Check sheet for the modelled part. Datum: model origin and axes. Units: mm. Give positions to 0.01 mm unless a question says otherwise; leave off trailing zeros. Write each loop counter-clockwise with the first axis right and the second up, starting at its lowest first coordinate (ties: lowest second). Pieces come first, ordered by that corner, then holes. Notation, with made-up numbers: M 30,38 L 69,38 A19 cw 69,74 Z; hole C -17,-5 d6. An arc over 180 degrees is marked long. One line per item, written item: value. Start each with the question number.
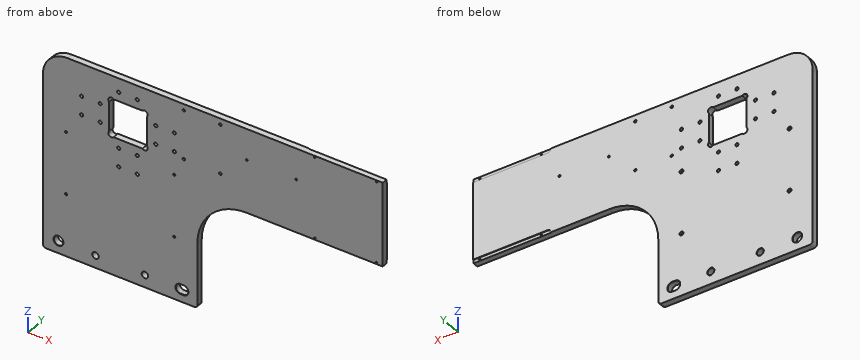
from build123d import *

# Parameters (mm, degrees)
SKETCH1_W                                      = 317.5
SKETCH1_H                                      = 406.4
BOSS_EXTRUDE1_DEPTH                            = 12.7
FILLET1_R                                      = 6.35
F_3_4_START                                    = 123.825
F_3_4_0_7500_DOWEL_SLOT1_3_DEPTH               = 6.35
F_1_2_CLEARANCE_HOLE1_D                        = 13.49248
F_1_2_CLEARANCE_HOLE1_CSINK_D                  = 14.76248
F_1_2_CLEARANCE_HOLE1_CSINK_ANGLE              = 90
SKETCH8_W                                      = 381
SKETCH8_H                                      = 171.45
BOSS_EXTRUDE2_DEPTH                            = 12.7
FILLET2_R                                      = 50.8
FILLET3_R                                      = 101.6
F_1_8_0_1250_DOWEL_HOLE1_D                     = 3.175
F_1_8_0_1250_DOWEL_HOLE1_CSINK_D               = 4.445
F_1_8_0_1250_DOWEL_HOLE1_CSINK_ANGLE           = 90
CUT_EXTRUDE1_DEPTH                             = 577.872249723
F_5_16_18_TAPPED_HOLE1_D                       = 6.5278
F_5_16_18_TAPPED_HOLE1_DEPTH                   = 20.1168
F_5_16_18_TAPPED_HOLE1_TIP                     = 1.961148974
CBORE_FOR_8_SOCKET_HEAD_CAP_SCREW1_D           = 4.4958
CBORE_FOR_8_SOCKET_HEAD_CAP_SCREW1_CBORE_D     = 7.9375
CBORE_FOR_8_SOCKET_HEAD_CAP_SCREW1_CBORE_DEPTH = 4.1656
SKETCH23_W                                     = 160.02
SKETCH23_H                                     = 6.858
CUT_EXTRUDE3_DEPTH                             = 1.27
FILLET4_R                                      = 6.35
F_10_32_TAPPED_HOLE1_D                         = 4.0386
F_1_4_20_TAPPED_HOLE1_D                        = 5.1054


with BuildPart() as part:
    # Sketch1 → Boss-Extrude1 (new body)
    with BuildSketch(Plane(origin=(0, 0, 0), x_dir=(1, 0, 0), z_dir=(0, 1, 0))):
        Rectangle(SKETCH1_W, SKETCH1_H)
    extrude(amount=BOSS_EXTRUDE1_DEPTH)

    # Fillet1
    fillet1_edges = [part.edges().sort_by_distance(p)[0] for p in [
        (-158.75, 6.35, -203.2),
        (158.75, 6.35, -203.2),
    ]]
    fillet(fillet1_edges, radius=FILLET1_R)

    # Sketch3 → 3/4 (0.7500) Dowel Hole1 (revolve, cut)
    with BuildSketch(Plane(origin=(-127, 12.7, -177.8), x_dir=(0, 0, 1), z_dir=(1, 0, 0))):
        Polygon((0, 0), (0, 12.7), (10.16, 12.7), (9.525, 12.065), (9.525, 0.635), (10.16, 0), align=None)
    revolve(axis=Axis((-127, 19.05, -177.8), (0, -1, 0)), mode=Mode.SUBTRACT)

    # 3/4 (0.7500) Dowel Slot1: read off the stored shape, not the designer's step
    # 3/4 (0.7500) Dowel Slot1 outline → 3/4 (0.7500) Dowel Slot1 (revolve, cut)
    with BuildSketch(Plane(origin=(130.175, 0, -177.8), x_dir=(1, 0, 0), z_dir=(0, 0, 1))):
        Polygon((0, 0), (10.16, 0), (9.525, 0.635), (9.525, 12.065), (10.16, 12.7), (0, 12.7), align=None)
    revolve(axis=Axis((130.175, 0, -177.8), (0, 1, 0)), mode=Mode.SUBTRACT)

    # 3_4 _0.7500_ Dowel Slot1 2 outline → 3_4 _0.7500_ Dowel Slot1 2 (revolve, cut)
    with BuildSketch(Plane(origin=(123.825, 0, -177.8), x_dir=(1, 0, 0), z_dir=(0, 0, 1))):
        Polygon((0, 0), (10.16, 0), (9.525, 0.635), (9.525, 12.065), (10.16, 12.7), (0, 12.7), align=None)
    revolve(axis=Axis((123.825, 0, -177.8), (0, 1, 0)), mode=Mode.SUBTRACT)

    # 3_4 _0.7500_ Dowel Slot1 3 outline → 3_4 _0.7500_ Dowel Slot1 3 (cut)
    with BuildSketch(Plane.YZ.offset(F_3_4_START)):
        Polygon((0.635, -187.325), (12.065, -187.325), (12.7, -187.96), (12.7, -167.64), (12.065, -168.275), (0.635, -168.275), (0, -167.64), (0, -187.96), align=None)
    extrude(amount=F_3_4_0_7500_DOWEL_SLOT1_3_DEPTH, mode=Mode.SUBTRACT)

    # 1/2 Clearance Hole1 (through all)
    with Locations(Plane(origin=(0, 12.7, 0), x_dir=(1, 0, 0), z_dir=(0, 1, 0))):
        with Locations((-50.8, 177.8), (50.8, 177.8)):
            CounterSinkHole(F_1_2_CLEARANCE_HOLE1_D / 2, F_1_2_CLEARANCE_HOLE1_CSINK_D / 2, counter_sink_angle=F_1_2_CLEARANCE_HOLE1_CSINK_ANGLE)

    # Sketch8 → Boss-Extrude2 (add)
    with BuildSketch(Plane(origin=(0, 0, 0), x_dir=(1, 0, 0), z_dir=(0, 1, 0))):
        with Locations((349.25, -117.475)):
            Rectangle(SKETCH8_W, SKETCH8_H)
    extrude(amount=BOSS_EXTRUDE2_DEPTH)

    # Fillet2
    fillet2_edges = [part.edges().sort_by_distance(p)[0] for p in [
        (-158.75, 6.35, 203.2),
    ]]
    fillet(fillet2_edges, radius=FILLET2_R)

    # Fillet3
    fillet3_edges = [part.edges().sort_by_distance(p)[0] for p in [
        (158.75, 6.35, 31.75),
    ]]
    fillet(fillet3_edges, radius=FILLET3_R)

    # 1/8 (0.1250) Dowel Hole1 (through all)
    with Locations(Plane(origin=(0, 12.7, 0), x_dir=(1, 0, 0), z_dir=(0, 1, 0))):
        with Locations((400.05, -34.925), (527.05, -34.925), (400.05, -200.025), (527.05, -200.025)):
            CounterSinkHole(F_1_8_0_1250_DOWEL_HOLE1_D / 2, F_1_8_0_1250_DOWEL_HOLE1_CSINK_D / 2, counter_sink_angle=F_1_8_0_1250_DOWEL_HOLE1_CSINK_ANGLE)

    # Sketch13 → Cut-Extrude1 (cut, through all)
    with BuildSketch(Plane(origin=(0, 12.7, 0), x_dir=(1, 0, 0), z_dir=(0, 1, 0))):
        with BuildLine():
            Line((-13.752743879, -156.21), (45.756743879, -156.21))
            ThreePointArc((45.756743879, -156.21), (54.737, -156.21), (54.737, -147.229743879))
            Line((54.737, -147.229743879), (54.737, -87.720256121))
            ThreePointArc((54.737, -87.720256121), (54.737, -78.74), (45.756743879, -78.74))
            Line((45.756743879, -78.74), (-13.752743879, -78.74))
            ThreePointArc((-13.752743879, -78.74), (-22.733, -78.74), (-22.733, -87.720256121))
            Line((-22.733, -87.720256121), (-22.733, -147.229743879))
            ThreePointArc((-22.733, -147.229743879), (-22.733, -156.21), (-13.752743879, -156.21))
        make_face()
    extrude(amount=-CUT_EXTRUDE1_DEPTH, mode=Mode.SUBTRACT)

    # 5/16-18 Tapped Hole1
    with Locations(Plane(origin=(0, 12.7, 0), x_dir=(1, 0, 0), z_dir=(0, 1, 0))):
        with Locations((-41.148, -98.425), (-41.148, -136.525), (73.152, -98.425), (73.152, -136.525), (-79.248, -98.425), (-79.248, -136.525), (111.252, -98.425), (111.252, -136.525), (-3.048, -60.325), (35.052, -60.325), (-3.048, -22.225), (35.052, -22.225), (-3.048, -174.625), (35.052, -174.625)):
            Hole(F_5_16_18_TAPPED_HOLE1_D / 2, depth=F_5_16_18_TAPPED_HOLE1_DEPTH)
            with Locations((0, 0, -(F_5_16_18_TAPPED_HOLE1_DEPTH + F_5_16_18_TAPPED_HOLE1_TIP / 2))):  # 118° drill point
                Cone(0, F_5_16_18_TAPPED_HOLE1_D / 2, F_5_16_18_TAPPED_HOLE1_TIP, mode=Mode.SUBTRACT)

    # CBORE for #8 Socket Head Cap Screw1 (through all)
    with Locations(Plane(origin=(0, 12.7, 0), x_dir=(1, 0, 0), z_dir=(0, 1, 0))):
        with Locations((-111.125, 76.2), (-111.125, -50.8), (111.125, 76.2), (111.125, -50.8)):
            CounterBoreHole(CBORE_FOR_8_SOCKET_HEAD_CAP_SCREW1_D / 2, CBORE_FOR_8_SOCKET_HEAD_CAP_SCREW1_CBORE_D / 2, CBORE_FOR_8_SOCKET_HEAD_CAP_SCREW1_CBORE_DEPTH)

    # Sketch23 → Cut-Extrude3 (cut)
    with BuildSketch(Plane(origin=(0, 12.7, 0), x_dir=(1, 0, 0), z_dir=(0, 1, 0))):
        with Locations((459.74, -35.179)):
            Rectangle(SKETCH23_W, SKETCH23_H)
        with Locations((459.74, -199.771)):
            Rectangle(SKETCH23_W, SKETCH23_H)
    extrude(amount=-CUT_EXTRUDE3_DEPTH, mode=Mode.SUBTRACT)

    # Fillet4
    fillet4_edges = [part.edges().sort_by_distance(p)[0] for p in [
        (379.73, 12.065, 38.608),
        (379.73, 12.065, 196.342),
    ]]
    fillet(fillet4_edges, radius=FILLET4_R)

    # #10-32 Tapped Hole1 (through all)
    with Locations(Plane(origin=(0, 12.7, 0), x_dir=(1, 0, 0), z_dir=(0, 1, 0))):
        with Locations((260.35, -139.7), (361.95, -139.7)):
            Hole(F_10_32_TAPPED_HOLE1_D / 2)

    # 1/4-20 Tapped Hole1 (through all)
    with Locations(Plane(origin=(0, 12.7, 0), x_dir=(1, 0, 0), z_dir=(0, 1, 0))):
        with Locations((130.937, -90.5), (205.937, -90.5), (205.937, -190.5), (130.937, -190.5)):
            Hole(F_1_4_20_TAPPED_HOLE1_D / 2)


solid = part.part
1) Gauge pin test, flat ends, axial feed: pin 1 (3.5 mm diameter, centred on x = 451, z = 198.5, fed in from +Y); pin 2 (2.5 mm diameter, centred on x = -112, z = 49.5, fed in from +Y); pin 3 (5 mm diameter, centred on x = -79.248, z = 136.525, fed in from +Y); pin 4 (0.6 mm diameter, centred on x = 427.5, y = 12.5, fed in from -Z). Record the tip position at first contact, or that the pin passes through.
2) Material ranges on L1, parallel to Z at x = 527.05, y = 2.5; L2, parallel to X at y = 6.5, z = 137; L3, parallel to Z at x = 111, y = 2, recorded low to high. Write a range as from..to.
3) Cross-section at A-A (z = -177.8). State how many separate pieces and enclosed holes the cut face has, plus the area to 3 significant figures.
4) Cross-section at B-B (x = 281). Record the boundary of the cut face in (y, z).
Data:
1. pin 1: stops at y = 11.43
1. pin 2: stops at y = 8.53
1. pin 3: passes through
1. pin 4: stops at z = 38.61
2. L1: z = 31.75..33.34, 36.51..198.44, 201.61..203.2
2. L2: x = -158.75..-82.48, -76.02..-44.38, -37.92..-22.73, 54.74..69.92, 76.38..108.02, 114.48..539.75
2. L3: z = -203.2..-78.44, -73.96..48.56, 53.04..95.17, 101.68..133.27, 139.78..203.2
3. separate pieces: 5
3. enclosed holes: 0
3. area: 3,120 mm2
4. outline: M 0,31.75 L 12.7,31.75 L 12.7,203.2 L 0,203.2 Z
